Autodesk Inventor part; units mm, degrees
ref_plane "YZ Plane" through (0, 0, 0) normal (1, 0, 0) x (0, 1, 0)
ref_plane "XZ Plane" through (0, 0, 0) normal (0, 1, 0) x (-1, 0, 0)
ref_plane "XY Plane" through (0, 0, 0) normal (0, 0, 1) x (1, 0, 0)
sketch "Sketch1" plane through (0, 0, 0) normal (0, 1, 0) x (-1, 0, 0)
  point P0 (0, 0)
sketch "Sketch2" plane through (0, 0, 0) normal (0, 1, 0) x (-1, 0, 0)
  line L0 (-0.2857, 31.4286) -> (-6.2857, 31.4286)
  line L1 (-6.2857, 31.4286) -> (-6.2857, -33.5714)
  line L2 (-6.2857, -33.5714) -> (-0.2857, -33.5714)
  line L3 (-0.2857, -33.5714) -> (-0.2857, 31.4286)
  line L4 (9.7143, -12.5714) -> (-0.2857, -12.5714)
  line L5 (-0.2857, -12.5714) -> (-0.2857, -33.5714)
  line L6 (-0.2857, -33.5714) -> (9.7143, -33.5714)
  line L7 (9.7143, -33.5714) -> (9.7143, -12.5714)
  point P0 (0, 0)
  point P1 (-0.2857, -12.5714)
  dimension "d0" = 44
  dimension "d1" = 6
  dimension "d2" = 10
  dimension "d3" = 65
extrude "Extrusion1" add sketch "Sketch2" along normal blind 1300
properties part number "UgolUkrep" material "Aluminum 6061"
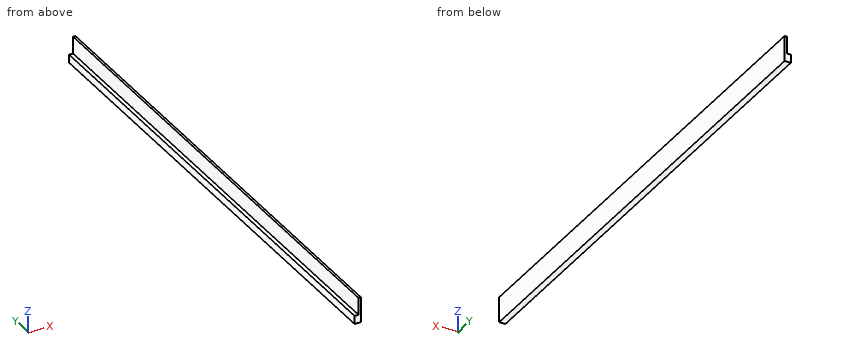
Can you work these out from the model? Positions are in its coordinate system, mm. Round coordinates to 2 decimals unless told otherwise and drop trailing zeros. Loops run counter-clockwise (first coordinate to the right, second up) from the corner with the lowest first, then second, coordinate; pieces in that order, holes last. Notation, with made-up numbers: (13.5, -21.5) - (58.5, -21.5) arc R19 cw to (58.5, -17.5) - close; hole circle Ø11 at (13, 62.5). An arc over 180 degrees is marked (long way). Use CSV: the item, a comma, the result in double quotes. Start each with the question number.
1) Please list where these lines run through material, in increasing order: probe 1 along Z at (x, y) = (-0.25, 1171); probe 2 along X at (y, z) = (604, 26.5). Write a range as [from, to].
2) If we section it at B-B on x = -6.25: Write out the boundary of the cut face in (y, z), plus the area to 3 significant figures.
3) If we section it at A-A on y = 233: Write out the boundary of the cut face in (x, z).
4) For pin 1 Ø12 at (y, z) = (766.5, -1.5) entering from -X; pin 2 Ø3 at (x, y) = (-4.5, 461) entering from +Z, each with a flat end and sliding along its axis, tell me the tip position at first contact or that it passes through.
5) If we section it at C-C on z = -1: Write out the boundary of the cut face in (x, y).
Geometry results:
1,probe 1,"z = [-33.57, -12.57]"
1,probe 2,"x = [0.29, 6.29]"
2,outline,"(0, -33.57) - (1300, -33.57) - (1300, -12.57) - (0, -12.57) - close"
2,area,"27,300 mm2"
3,outline,"(-9.71, -33.57) - (6.29, -33.57) - (6.29, 31.43) - (0.29, 31.43) - (0.29, -12.57) - (-9.71, -12.57) - close"
4,pin 1,"stops at x = 0.29"
4,pin 2,"stops at z = -12.57"
5,outline,"(0.29, 0) - (6.29, 0) - (6.29, 1300) - (0.29, 1300) - close"
